Read the model definition and answer for the solid it produces. Units are mm, in the model's axes. Give positions to 0.01 mm unless a question says otherwise; leave off trailing zeros. Order: outer loops, then holes, each group sorted by start corner. A loop starts at its lowest first (then second) coordinate and runs counter-clockwise, first axis right, second up. Notation, with made-up numbers: (52.5, -29) - (62.5, -29) arc R21 ccw to (62.5, 7) - close; hole circle Ø9 at (3, -19.75). An arc over 180 degrees is marked (long way). Write item = value, one per line.
Autodesk Fusion 360 part; units mm, degrees
sketch "Sketch1" plane through (0, 0, 0) normal (0, 0, 1) x (1, 0, 0)
  line L0 (0, 0) -> (0, 100)
  line L1 (0, 100) -> (40, 100)
  line L2 (40, 100) -> (100, 0)
  line L3 (100, 0) -> (0, 0)
  circle A0 centre (30, 12.5) radius 2.55
  circle A1 centre (60, 12.5) radius 2.55
  dimension "d3" = 40
  dimension "d4" = 100
  dimension "d5" = 100
  dimension "d14" = 12.5
  dimension "d15" = 12.5
  dimension "d16" = 5.1
  dimension "d17" = 5.1
  dimension "d18" = 30
  dimension "d19" = 30
extrude "Extrude1" add sketch "Sketch1" along normal blind 8.5
equation "d15 = d14"
equation "d17 = d16"
1. Section C-C (z = 1.25) is taken. Determine the outline of the cut face in (x, y).
Recorded:
outline = (0, 0) - (100, 0) - (40, 100) - (0, 100) - close; hole circle Ø5.1 at (30, 12.5); hole circle Ø5.1 at (60, 12.5)
2. Section B-B (x = 30) is taken. Determine the outline of the cut face in (y, z).
Recorded:
outline = (0, 0) - (9.95, 0) - (9.95, 8.5) - (0, 8.5) - close; (15.05, 0) - (100, 0) - (100, 8.5) - (15.05, 8.5) - close
3. Section A-A (y = 12.5) is taken. Determine the outline of the cut face in (x, z), and give its area (3 significant figures).
Recorded:
outline = (0, 0) - (27.45, 0) - (27.45, 8.5) - (0, 8.5) - close; (32.55, 0) - (57.45, 0) - (57.45, 8.5) - (32.55, 8.5) - close; (62.55, 0) - (92.5, 0) - (92.5, 8.5) - (62.55, 8.5) - close
area = 700 mm^2
4. A flat-ended cylindrical pin translates along its axis: pin 1 (2 mm diameter, centred on x = 66, y = 59, fed in from +Z). Find the tip coordinate at first contact, or state that the pin passes through.
Recorded:
pin_1 = through
5. Straight lines are drawn through the part: L1, parallel to Y at x = 30, z = 6.5; L2, parallel to Y at x = 60, z = 6.75; L3, parallel to Y at x = 53, z = 4.75. For each, find the intervals that lie inside material, in ascending order. Write a range as [from, to].
Recorded:
L1 = [0, 9.95], [15.05, 100]
L2 = [0, 9.95], [15.05, 66.67]
L3 = [0, 78.33]
6. Determine the mould class of faces 1 (the face through (57.452, 12.388, 4.19)), 2 (the face through (27.452, 12.388, 4.19)), 3 (the face through (69.58, 50.7, 4.19)), 4 (the face through (38, 40, 0)) for opening direction Y: +Y half, -Y half, draft (parallel to the pull), parting line (faces both ways), or undercut.
Recorded:
face_1 = undercut
face_2 = undercut
face_3 = +Y half
face_4 = draft
7. Section D-D (y = 54.5) is taken. Determine the outline of the cut face in (x, z), and give its area (3 significant figures).
Recorded:
outline = (0, 0) - (67.3, 0) - (67.3, 8.5) - (0, 8.5) - close
area = 572 mm^2
